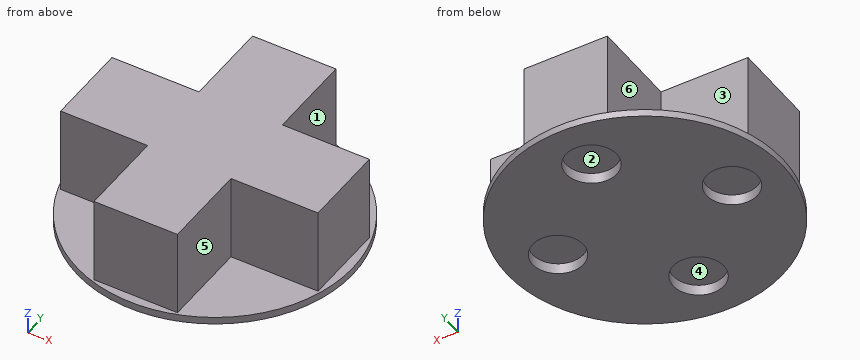
from build123d import *

# Parameters (mm, degrees)
BOSS_EXTRUDE1_DEPTH = 6
SKETCH2_R           = 9.5
BOSS_EXTRUDE2_DEPTH = 0.5
SKETCH4_R           = 1.75
CUT_EXTRUDE2_DEPTH  = 0.75


with BuildPart() as part:
    # Sketch1 → Boss-Extrude1 (new body)
    with BuildSketch(Plane.XY):
        Polygon((-2.875, 2.875), (-2.875, 8.875), (2.875, 8.875), (2.875, 2.875), (8.875, 2.875), (8.875, -2.875), (2.875, -2.875), (2.875, -8.875), (-2.875, -8.875), (-2.875, -2.875), (-8.875, -2.875), (-8.875, 2.875), align=None)
    extrude(amount=BOSS_EXTRUDE1_DEPTH)

    # Sketch2 → Boss-Extrude2 (add)
    with BuildSketch(Plane(origin=(0, 0, 0), x_dir=(-1, 0, 0), z_dir=(0, 0, -1))):
        Circle(SKETCH2_R)
    extrude(amount=BOSS_EXTRUDE2_DEPTH)

    # Sketch4 → Cut-Extrude2 (cut)
    with BuildSketch(Plane(origin=(0, 0, -0.5), x_dir=(-1, 0, 0), z_dir=(0, 0, -1))):
        with Locations((6, 0)):
            Circle(SKETCH4_R)
        with Locations((0, -6)):
            Circle(SKETCH4_R)
        with Locations((-6, 0)):
            Circle(SKETCH4_R)
        with Locations((0, 6)):
            Circle(SKETCH4_R)
    extrude(amount=-CUT_EXTRUDE2_DEPTH, mode=Mode.SUBTRACT)


solid = part.part
Work out the finished part from the listing and answer in its coordinate system (mm). Face numbers are marked on the shaded views. A direction names the side the tool comes from. Round coordinates to 2 decimals unless told otherwise and drop trailing zeros. Order: outer loops, then holes, each group sorted by start corner. A loop starts at its lowest first (then second) coordinate and runs counter-clockwise, first axis right, second up. Notation, with made-up numbers: M 25,78.5 L 73,78.5 A11 cw 73,83.5 Z; hole C 58,6 d1. An arc over 180 degrees is marked long. Put each result on its own line as item: value. Start each with the question number.
Q1. Section A-A, the plane z = 4 is taken. Write down the section's boundary in (x, y) (3 decimals), and give its area (3 significant figures).
Q2. For a pull along X with two mould halves and no side action, classify the marked faces 1, 2 and 3 as pulls with the +X half, pulls with the -X half, needs draft (parallel to the pull), parting line crosses it, or undercut.
Q3. Flat-ended cylindrical pins translate along their axes: pin 1 (1.8 mm diameter, centred on x = -5.5, y = -0.5, fed in from -Z); pin 2 (2 mm diameter, centred on x = -6, z = 4.5, fed in from +Y) (3 decimals); pin 3 (3 mm diameter, centred on y = -5, z = 2.5, fed in from -X) (3 decimals); pin 4 (3 mm diameter, centred on x = 0.5, y = 6, fed in from -Z). Find the tip coordinate at first contact, or state that the pin passes through.
Q4. Section D-D, the plane x = -3.5 is taken. Write down the section's boundary in (y, z) (3 decimals).
Q5. Section B-B, the plane y = 0 is taken. Write down the section's boundary in (x, z) (3 decimals), and give its area (3 significant figures).
Q6. A tool of negligible diameter and unlimited length cuts with its end or side. For the marked faces 4, 5 and 6, from which of +Z, -Z, +X, -X, +Y, -Y can it reach the whole face along a straight path? Write none if from no direction.
Q7. Straight lines are drawn through the part: L1, parallel to Y at x = 0, z = -0.15; L2, parallel to X at y = 8.25, z = 2.5 (3 decimals); L3, parallel to X at y = -1.5, z = 1 (3 decimals). For each, find the intervals that lie inside material, in ascending order. Write a range as [from, to].
Findings below:
1. outline: M -8.875,-2.875 L -2.875,-2.875 L -2.875,-8.875 L 2.875,-8.875 L 2.875,-2.875 L 8.875,-2.875 L 8.875,2.875 L 2.875,2.875 L 2.875,8.875 L -2.875,8.875 L -2.875,2.875 L -8.875,2.875 Z
1. area: 171 mm^2
2. face 1: pulls with the +X half
2. face 2: undercut
2. face 3: needs draft
3. pin 1: stops at z = 0.25
3. pin 2: stops at y = 2.875
3. pin 3: stops at x = -2.875
3. pin 4: stops at z = -0.5
4. outline: M -8.832,-0.5 L 8.832,-0.5 L 8.832,0 L 2.875,0 L 2.875,6 L -2.875,6 L -2.875,0 L -8.832,0 Z
5. outline: M -9.5,-0.5 L -7.75,-0.5 L -7.75,0.25 L -4.25,0.25 L -4.25,-0.5 L 4.25,-0.5 L 4.25,0.25 L 7.75,0.25 L 7.75,-0.5 L 9.5,-0.5 L 9.5,0 L 8.875,0 L 8.875,6 L -8.875,6 L -8.875,0 L -9.5,0 Z
5. area: 111 mm^2
6. face 4: -Z
6. face 5: +Z, +X, -Y
6. face 6: +Z, -X, +Y
7. L1: y = [-9.5, -7.75], [-4.25, 4.25], [7.75, 9.5]
7. L2: x = [-2.875, 2.875]
7. L3: x = [-8.875, 8.875]
